Work out the finished part from the listing and answer in its coordinate system (mm). A direction names the side the tool comes from. Round coordinates to 2 decimals unless told otherwise and drop trailing zeros. Loops run counter-clockwise (first coordinate to the right, second up) from the corner with the lowest first, then second, coordinate; pieces in that order, holes last.
```python
from build123d import *

# Parameters (mm, degrees)
SKETCH1_W           = 65
SKETCH1_H           = 5
SKETCH1_R           = 1.5
BOSS_EXTRUDE1_DEPTH = 3
SKETCH2_R           = 2.5
SKETCH2_R_2         = 1.5
BOSS_EXTRUDE2_DEPTH = 22
FILLET1_R           = 3


with BuildPart() as part:
    # Sketch1 → Boss-Extrude1 (new body)
    with BuildSketch(Plane(origin=(0, 0, 0), x_dir=(1, 0, 0), z_dir=(0, 1, 0))):
        with Locations((32.5, 2.5)):
            Rectangle(SKETCH1_W, SKETCH1_H)
        with Locations(Location((5, 2.5, 0), (0, 0, 270))):
            Circle(SKETCH1_R, mode=Mode.SUBTRACT)
        with Locations(Location((10, 2.5, 0), (0, 0, 270))):
            Circle(SKETCH1_R, mode=Mode.SUBTRACT)
        with Locations(Location((15, 2.5, 0), (0, 0, 270))):
            Circle(SKETCH1_R, mode=Mode.SUBTRACT)
        with Locations(Location((20, 2.5, 0), (0, 0, 270))):
            Circle(SKETCH1_R, mode=Mode.SUBTRACT)
        with Locations(Location((25, 2.5, 0), (0, 0, 270))):
            Circle(SKETCH1_R, mode=Mode.SUBTRACT)
        with Locations(Location((30, 2.5, 0), (0, 0, 270))):
            Circle(SKETCH1_R, mode=Mode.SUBTRACT)
        with Locations(Location((35, 2.5, 0), (0, 0, 270))):
            Circle(SKETCH1_R, mode=Mode.SUBTRACT)
        with Locations(Location((40, 2.5, 0), (0, 0, 270))):
            Circle(SKETCH1_R, mode=Mode.SUBTRACT)
        with Locations(Location((45, 2.5, 0), (0, 0, 270))):
            Circle(SKETCH1_R, mode=Mode.SUBTRACT)
        with Locations(Location((50, 2.5, 0), (0, 0, 270))):
            Circle(SKETCH1_R, mode=Mode.SUBTRACT)
        with Locations(Location((55, 2.5, 0), (0, 0, 270))):
            Circle(SKETCH1_R, mode=Mode.SUBTRACT)
        with Locations(Location((60, 2.5, 0), (0, 0, 270))):
            Circle(SKETCH1_R, mode=Mode.SUBTRACT)
    extrude(amount=BOSS_EXTRUDE1_DEPTH)

    # Sketch2 → Boss-Extrude2 (add)
    # profile 1 of 2: a face of its own
    with BuildSketch(Plane(origin=(0, 3, 0), x_dir=(1, 0, 0), z_dir=(0, 1, 0))):
        with Locations(Location((5, 2.5, 0), (0, 0, 270))):
            Circle(SKETCH2_R)
        with Locations(Location((5, 2.5, 0), (0, 0, 270))):
            Circle(SKETCH2_R_2, mode=Mode.SUBTRACT)
    # profile 2 of 2: a face of its own
    with BuildSketch(Plane(origin=(0, 3, 0), x_dir=(1, 0, 0), z_dir=(0, 1, 0))):
        with Locations(Location((60, 2.5, 0), (0, 0, 270))):
            Circle(SKETCH2_R)
        with Locations(Location((60, 2.5, 0), (0, 0, 270))):
            Circle(SKETCH2_R_2, mode=Mode.SUBTRACT)
    extrude(amount=BOSS_EXTRUDE2_DEPTH)

    # Fillet1
    # the kernel refuses this fillet: 3 mm, written as the material it takes off along each edge
    with BuildSketch(Plane(origin=(65, -7.5, -5), x_dir=(-1, 0, 0), z_dir=(0, 1, 0)), Plane(origin=(0, -7.5, 0), x_dir=(1, 0, 0), z_dir=(0, 1, 0))) as fillet1_piece_1:
        with BuildLine():
            CenterArc((FILLET1_R, FILLET1_R), FILLET1_R, 180, 90)
            Line((0, FILLET1_R), (0, 0))
            Line((0, 0), (FILLET1_R, 0))
        make_face()
    extrude(amount=18, mode=Mode.SUBTRACT)
    with BuildSketch(Plane(origin=(65, -7.5, 0), x_dir=(-1, 0, 0), z_dir=(0, 1, 0)), Plane(origin=(0, -7.5, -5), x_dir=(1, 0, 0), z_dir=(0, 1, 0))) as fillet1_piece_2:
        with BuildLine():
            CenterArc((FILLET1_R, -FILLET1_R), FILLET1_R, 90, 90)
            Line((0, -FILLET1_R), (0, 0))
            Line((0, 0), (FILLET1_R, 0))
        make_face()
    extrude(amount=18, mode=Mode.SUBTRACT)


solid = part.part
```
1. Given pin 1 (2.5 mm diameter, centred on x = 55, z = -2.5, fed in from +Y); pin 2 (1.5 mm diameter, centred on x = 2, z = -1.5, fed in from +Y); pin 3 (1.5 mm diameter, centred on x = 32.5, z = -3, fed in from +Y), each flat-ended and moving along its own axis, determine where each tip first touches the part or whether it passes through.
Answer key:
pin 1: passes through
pin 2: stops at y = 25
pin 3: stops at y = 3
2. Find section B-B (x = 30). Write down the section's boundary in (y, z), then the cut area to 3 significant figures.
Answer key:
outline: (0, -5) - (3, -5) - (3, -4) - (0, -4) - close; (0, -1) - (3, -1) - (3, 0) - (0, 0) - close
area: 6.00 mm2
3. Find section A-A (y = 15). Write down the section's boundary in (x, z), then the cut area to 3 significant figures.
Answer key:
outline: circle Ø5 at (5, -2.5); circle Ø5 at (60, -2.5); hole circle Ø3 at (5, -2.5); hole circle Ø3 at (60, -2.5)
area: 25.1 mm2
4. Which of the six approach directions +Z, -Z, +X, -X, +Y, -Y give full straight-line access (tool end or side, diameter ignored) to faces 1 (the face through (63, 3, -3)), 2 (the face through (1.04, 1.48, -0.73)), 3 (the face through (7.48, 13.85, -2.83))?
Answer key:
face 1: +X, +Y
face 2: +Z, -X, +Y, -Y
face 3: +Y
5. Consider probe 1 along X at (y, z) = (4.5, -3.1); probe 2 along X at (y, z) = (10, -1.4) (3 decimals); probe 3 along Y at (x, z) = (45.5, -4.75). Determine where each line is inside the solid, lowest interval first.
Answer key:
probe 1: x = 2.57 to 3.63, 6.37 to 7.43, 57.57 to 58.63, 61.37 to 62.43
probe 2: x = 2.755 to 3.98, 6.02 to 7.245, 57.755 to 58.98, 61.02 to 62.245
probe 3: y = 0 to 3
6. Determine the mould class of faces 4 (the face through (57.56, 13.85, -3.04)), 5 (the face through (26.487, 1.479, -2.695)), 6 (the face through (1.086, 1.479, -4.31)) for opening direction Z: +Z half, -Z half, draft (parallel to the pull), parting line (faces both ways), or undercut.
Answer key:
face 4: parting line
face 5: undercut
face 6: -Z half
7. Find section C-C (x = 17.5). Write down the section's boundary in (y, z), then the cut area to 3 significant figures.
Answer key:
outline: (0, -5) - (3, -5) - (3, 0) - (0, 0) - close
area: 15.0 mm2
